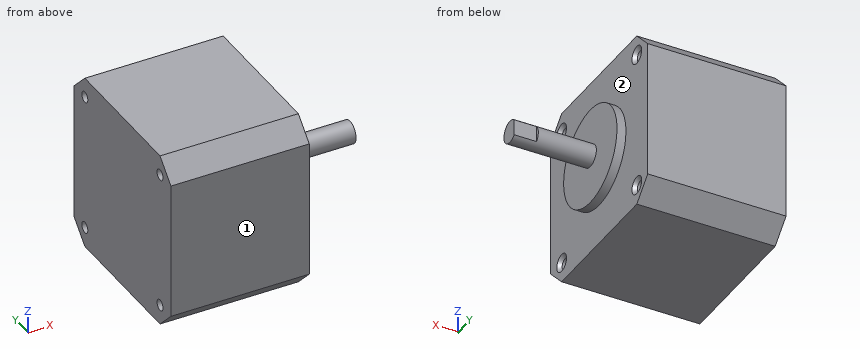
Autodesk Inventor part; units mm, degrees
ref_plane "YZ Plane" through (0, 0, 0) normal (1, 0, 0) x (0, 1, 0)
ref_plane "XZ Plane" through (0, 0, 0) normal (0, 1, 0) x (-1, 0, 0)
ref_plane "XY Plane" through (0, 0, 0) normal (0, 0, 1) x (1, 0, 0)
sketch "Sketch1" plane through (0, 0, 0) normal (1, 0, 0) x (0, 1, 0)
  line L0 (-20, 20) -> (20, 20)
  line L1 (20, 20) -> (20, -20)
  line L2 (20, -20) -> (-20, -20)
  line L3 (-20, -20) -> (-20, 20)
  line L4 (-20, 20) -> (20, -20) construction
  line L5 (20, 20) -> (-20, -20) construction
  point P0 (0, 0)
  point P1 (0, 0)
  dimension "d0" = 40
  dimension "d1" = 40
extrude "Extrusion1" add sketch "Sketch1" along normal blind 33
sketch "Sketch2" plane through (33, 0, 0) normal (1, 0, 0) x (0, 0, -1)
  line L0 (-20, 20) -> (-20, -20)
  line L1 (-20, -20) -> (20, -20)
  line L2 (20, -20) -> (20, 20)
  line L3 (20, 20) -> (-20, 20)
  circle A0 centre (0, 0) radius 11
  dimension "d4" = 22
extrude "Extrusion2" cut sketch "Sketch2" against normal blind 2
sketch "Sketch3" plane through (33, 0, 0) normal (1, 0, 0) x (0, 0, -1)
  circle A0 centre (0, 0) radius 2.5
  dimension "d7" = 5
extrude "Extrusion3" add sketch "Sketch3" along normal blind 18
sketch "Sketch4" plane through (31, 0, 0) normal (1, 0, 0) x (0, 0, -1)
  line L0 (20, 20) -> (20, -20)
  line L1 (-20, 20) -> (20, 20)
  point P0 (15.5, 15.5)
  point P1 (-15.5, 15.5)
  point P2 (15.5, -15.5)
  point P3 (-15.5, -15.5)
  dimension "d12" = 31
  dimension "d15" = 31
hole "Hole1" at (31, 15.5, -15.5) at (31, 15.5, 15.5) at (31, -15.5, -15.5) at (31, -15.5, 15.5) direction (-1, 0, 0) diameter 2.459 end through all countersink diameter 4 countersink angle 90
chamfer "Chamfer1" distance 4.5 angle 45 4 edges at (15.5, 20, -20) (15.5, -20, -20) (15.5, 20, 20) (15.5, -20, 20)
sketch "Sketch7" plane through (51, 0, 0) normal (1, 0, 0) x (0, 0, -1)
  line L0 (-2.5, 1.7499) -> (2.5, 1.7499)
  line L1 (2.5, 1.7499) -> (2.5, 3.2499)
  line L2 (2.5, 3.2499) -> (-2.5, 3.2499)
  line L3 (-2.5, 3.2499) -> (-2.5, 1.7499)
  line L4 (-2.5, 1.7499) -> (2.5, 3.2499) construction
  line L5 (2.5, 1.7499) -> (-2.5, 3.2499) construction
  point P0 (0, 2.4999)
  dimension "d29" = 5
  dimension "d30" = 1.5
extrude "Extrusion4" cut sketch "Sketch7" against normal blind 5
properties part number "Stepper_Motor"
The listing builds one solid part. Answer for the finished solid, in the listing's coordinates (mm). Face numbers are marked on the shaded views. A direction names the side the tool comes from. Round coordinates to 2 decimals unless told otherwise and drop trailing zeros. Order: outer loops, then holes, each group sorted by start corner. A loop starts at its lowest first (then second) coordinate and runs counter-clockwise, first axis right, second up. Notation, with made-up numbers: (25.25, -24.5) -> (49.25, -24.5) arc R14 ccw to (49.25, -7.5) -> close; hole circle Ø10 at (13, -27.75). An arc over 180 degrees is marked (long way). Answer as CSV lines item,"result". Start each with the question number.
(1) A tool of negligible diameter and unlimited length cuts with its end or side. For the marked faces 1 and 2, from which of +Z, -Z, +X, -X, +Y, -Y can it reach the whole face along a straight path? Write none if from no direction.
(2) Find the intervals of material crossed by probe 1 along Y at (x, z) = (17, 15.5); probe 2 along Y at (x, z) = (19, 15), in increasing order. Write a range as from..to.
(3) Flat-ended cylindrical pins translate along their axes: pin 1 Ø3 at (x, z) = (48.5, 0) entering from +Y; pin 2 Ø2 at (x, y) = (35, -12) entering from -Z; pin 3 Ø6 at (y, z) = (7.5, 1) entering from +X; pin 4 Ø1.5 at (y, z) = (16, -0.5) entering from +X. Find the tip coordinate at first contact, or state that the pin passes through.
(4) The part is cut by section D-D (z = -5.5). Determine the outline of the cut face in (x, y).
(5) The part is cut by section A-A (x = 29.5). Determine the outline of the cut face in (y, z).
(6) The part is cut by section C-C (y = -6). Determine the outline of the cut face in (x, z), then the cut area to 3 significant figures.
(7) The part is cut by section B-B (z = 0). Determine the outline of the cut face in (x, y).
Evaluation:
1,face 1,"+Z, -Z, +X, -X, -Y"
1,face 2,"+X"
2,probe 1,"-20..-16.73, -14.27..14.27, 16.73..20"
2,probe 2,"-20..-16.62, -14.38..14.38, 16.62..20"
3,pin 1,"y = 1.75"
3,pin 2,"through"
3,pin 3,"x = 33"
3,pin 4,"x = 31"
4,outline,"(0, -20) -> (31, -20) -> (31, -9.53) -> (33, -9.53) -> (33, 9.53) -> (31, 9.53) -> (31, 20) -> (0, 20) -> close"
5,outline,"(-20, -15.5) -> (-15.5, -20) -> (15.5, -20) -> (20, -15.5) -> (20, 15.5) -> (15.5, 20) -> (-15.5, 20) -> (-20, 15.5) -> close; hole circle Ø2.46 at (-15.5, -15.5); hole circle Ø2.46 at (-15.5, 15.5); hole circle Ø2.46 at (15.5, -15.5); hole circle Ø2.46 at (15.5, 15.5)"
6,outline,"(0, -20) -> (31, -20) -> (31, -9.22) -> (33, -9.22) -> (33, 9.22) -> (31, 9.22) -> (31, 20) -> (0, 20) -> close"
6,area,"1,280 mm²"
7,outline,"(0, -20) -> (31, -20) -> (31, -11) -> (33, -11) -> (33, -2.5) -> (51, -2.5) -> (51, 1.75) -> (46, 1.75) -> (46, 2.5) -> (33, 2.5) -> (33, 11) -> (31, 11) -> (31, 20) -> (0, 20) -> close"
